Autodesk Inventor part; units mm, degrees
ref_plane "YZ Plane" through (0, 0, 0) normal (1, 0, 0) x (0, 1, 0)
ref_plane "XZ Plane" through (0, 0, 0) normal (0, 1, 0) x (-1, 0, 0)
ref_plane "XY Plane" through (0, 0, 0) normal (0, 0, 1) x (1, 0, 0)
sketch "Sketch2" plane through (0, 0, 0) normal (0, 1, 0) x (-1, 0, 0)
  line L0 (105, -2) -> (-105, -2)
  line L1 (-105, -2) -> (-105, 2)
  line L2 (-105, 2) -> (105, 2)
  line L3 (105, 2) -> (105, -2)
  line L4 (105, -2) -> (-105, 2) construction
  line L5 (-105, -2) -> (105, 2) construction
  point P0 (0, 0)
  dimension "d1" = 210
  dimension "d2" = 4
extrude "Extrusion1" add sketch "Sketch2" along normal blind 100
sketch "Sketch3" plane through (-105, 0, 2) normal (0, 0, 1) x (1, 0, 0)
  line L0 (0, 0) -> (0, 100)
  line L1 (0, 20) -> (210, 50)
  line L2 (210, 0) -> (210, 100)
  line L3 (0, 0) -> (210, 0)
  line L4 (0, 0) -> (210, 0)
  line L5 (210, 0) -> (210, 100)
  line L6 (0, 100) -> (210, 100)
  line L7 (0, 0) -> (0, 100)
  point P0 (105, 0)
  dimension "d5" = 20
  dimension "d37" = 30
extrude "Extrusion2" cut sketch "Sketch3" against normal up to next contours L0 L6 L2 L1
sketch "Sketch4" plane through (0, 0, 0) normal (0, -1, 0) x (1, 0, 0)
  line L0 (105, 2) -> (55, 2)
  line L1 (55, 2) -> (55, -2)
  line L2 (55, -2) -> (105, -2)
  line L3 (105, -2) -> (105, 2)
  line L4 (-105, 2) -> (105, 2)
  line L5 (-105, -2) -> (-105, 2)
  line L6 (105, -2) -> (-105, -2)
  line L7 (105, 2) -> (105, -2)
  line L8 (55, 2) -> (5, 2)
  line L9 (5, 2) -> (5, -2)
  line L10 (5, -2) -> (55, -2)
  line L11 (55, -2) -> (55, 2)
  line L12 (5, 2) -> (-45, 2)
  line L13 (-45, 2) -> (-45, -2)
  line L14 (-45, -2) -> (5, -2)
  line L15 (5, -2) -> (5, 2)
  line L16 (-45, 2) -> (-95, 2)
  line L17 (-95, 2) -> (-95, -2)
  line L18 (-95, -2) -> (-45, -2)
  line L19 (-45, -2) -> (-45, 2)
  point P0 (0, 0)
  point P1 (55, -2)
  point P2 (5, -2)
  point P3 (-45, -2)
  dimension "d9" = 50
  dimension "d10" = 4
  dimension "d13" = 50
extrude "Extrusion3" add sketch "Sketch4" along normal blind 4 contours L3 L2 L1 L0 | L9 L6 L13 L4 | L17 L6 L5 L4
sketch "Sketch5" plane through (-95, 0, 2) normal (0, 0, 1) x (1, 0, 0)
  line L0 (-10, 20) -> (-10, -4)
  line L1 (0, -4) -> (-10, -4)
  line L2 (0, 0) -> (0, -4)
  line L3 (0, 0) -> (50, 0)
  line L4 (50, 0) -> (50, -4)
  line L5 (100, -4) -> (50, -4)
  line L6 (100, 0) -> (100, -4)
  line L7 (100, 0) -> (150, 0)
  line L8 (150, 0) -> (150, -4)
  line L9 (200, -4) -> (150, -4)
  line L10 (200, -4) -> (200, 50)
  line L11 (200, 50) -> (-10, 20)
  line L12 (-5, 15.6635) -> (192.9899, 43.9478)
  line L13 (19.7487, 19.1991) -> (69.2462, 26.2701)
  line L14 (69.2462, 26.2701) -> (69.8119, 22.3103)
  line L15 (69.8119, 22.3103) -> (20.3144, 15.2393)
  line L16 (20.3144, 15.2393) -> (19.7487, 19.1991)
  line L17 (118.7437, 33.3412) -> (119.3094, 29.3814)
  line L18 (69.8119, 22.3103) -> (69.2462, 26.2701)
  line L19 (119.3094, 29.3814) -> (69.8119, 22.3103)
  line L20 (69.2462, 26.2701) -> (118.7437, 33.3412)
  line L21 (168.2412, 40.4123) -> (168.8068, 36.4525)
  line L22 (119.3094, 29.3814) -> (118.7437, 33.3412)
  line L23 (168.8068, 36.4525) -> (119.3094, 29.3814)
  line L24 (118.7437, 33.3412) -> (168.2412, 40.4123)
  line L25 (200, 50) -> (-10, 20)
  point P0 (95, 0)
  point P1 (200, 100)
  point P2 (168.2412, 40.4123)
  dimension "d20" = 200
  dimension "d24" = 4
  dimension "d25" = 50
  dimension "d26" = 5
  dimension "d27" = 25
  dimension "d30" = 50
extrude "Extrusion4" cut sketch "Sketch5" against normal up to next contours L12 L14 L15 L16 | L12 L21 L23 L17
properties part number "ControlPanelSide_V1"
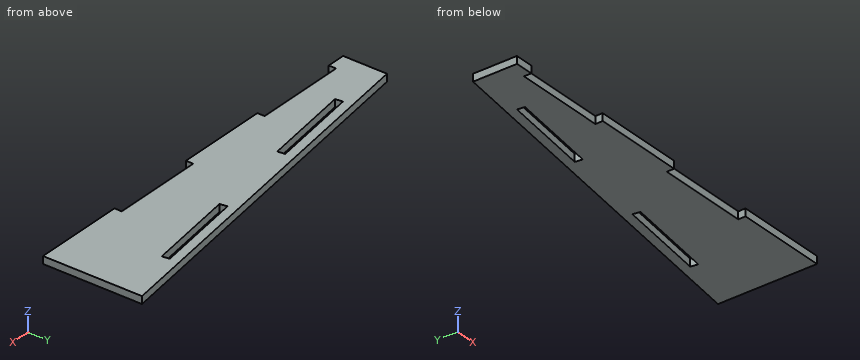
Read the model definition and answer for the solid it produces. Units are mm, in the model's axes. Round coordinates to 2 decimals unless told otherwise and drop trailing zeros. Write each loop counter-clockwise with the first axis right and the second up, starting at its lowest first coordinate (ties: lowest second). Pieces come first, ordered by that corner, then holes. Notation, with made-up numbers: M 7.5,-24.75 L 25.5,-24.75 A31 cw 25.5,9.25 Z; hole C 20,69 d7. An arc over 180 degrees is marked long. One line per item, written item: value.
Q1. Find section B-B on x = -53.5. Write down the section's boundary in (y, z), plus the area to 3 significant figures.
Data:
outline: M 0,-2 L 18.27,-2 L 18.27,2 L 0,2 Z; M 22.31,-2 L 27.36,-2 L 27.36,2 L 22.31,2 Z
area: 93.3 mm2
Q2. Find section D-D on x = 53. Write down the section's boundary in (y, z).
Data:
outline: M 0,-2 L 33.48,-2 L 33.48,2 L 0,2 Z; M 37.52,-2 L 42.57,-2 L 42.57,2 L 37.52,2 Z
Q3. Find section C-C on y = 47.5. Write down the section's boundary in (x, z).
Data:
outline: M 87.5,-2 L 105,-2 L 105,2 L 87.5,2 Z
Q4. Find section A-A on z = 0.25. Write down the section's boundary in (x, y), plus the area to 3 significant figures.
Data:
outline: M -105,-4 L -95,-4 L -95,0 L -45,0 L -45,-4 L 5,-4 L 5,0 L 55,0 L 55,-4 L 105,-4 L 105,50 L -105,20 Z; hole M -75.25,19.2 L -74.69,15.24 L -25.19,22.31 L -25.75,26.27 Z; hole M 23.74,33.34 L 24.31,29.38 L 73.81,36.45 L 73.24,40.41 Z
area: 7,390 mm2
Q5. Flat-ended cylindrical pins translate along their axes: pin 1 Ø2 at (x, z) = (27.5, -0.5) entering from -Y; pin 2 Ø1.5 at (x, z) = (30.5, -1.5) entering from +Y. Find the tip coordinate at first contact, or state that the pin passes through.
Data:
pin 1: y = 0
pin 2: y = 39.46
Q6. Straight lines are drawn through the part: line 1 (X direction, y = -0.5, z = -1); line 2 (Y direction, x = 35, z = -0.85); line 3 (Y direction, x = -45.5, z = -0.4). For each, find the intervals that lie inside material, in ascending order. Write a range as [from, to].
Data:
line 1: [-105, -95], [-45, 5], [55, 105]
line 2: [0, 30.91], [34.95, 40]
line 3: [0, 19.41], [23.45, 28.5]
